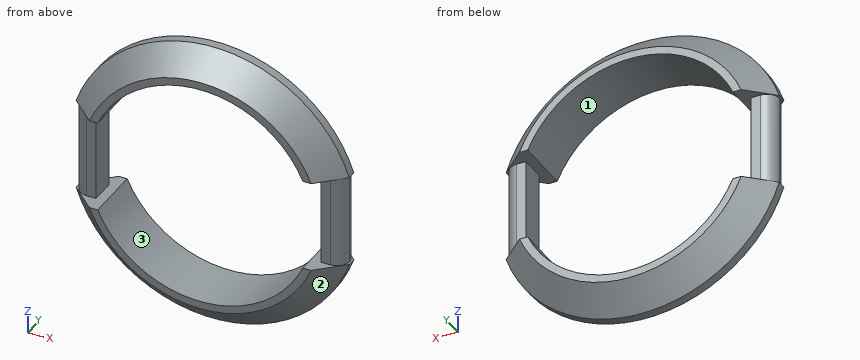
from build123d import *

# Parameters (mm, degrees)
F1_DEPTH      = 2.25
F1_DEPTH_BACK = 2.25
F2_DEPTH      = 1
F2_DEPTH_BACK = 1
F3_T2_ANGLE   = 191.9949180636
F3_T4_ANGLE   = 191.9949180636
F3_T6_ANGLE   = 191.9949180636
F3_T8_ANGLE   = 191.9949180636
F4_T4_DEPTH   = 11.4223278392
F4_T10_DEPTH  = 11.4223278392
F4_T16_DEPTH  = 11.4223278392
F4_T22_DEPTH  = 11.4223278392


# Not quite as in the source:
# - a fillet or chamfer that OpenCascade refuses, or shapes differently, is made with other operations: its cross-section is extruded or revolved along the edge and cut away or added


with BuildPart() as f1:
    # F0 (on Front) → F1 (new body, two sides)
    with BuildSketch(Plane.XZ) as f1_sk:
        with BuildLine():
            ThreePointArc((-8.0962065927, 3.6355279959), (0, 8.875), (8.0962065927, 3.6355279959))
            Line((8.0962065927, 3.6355279959), (8.875, 3.6355279959))
            Line((8.875, 3.6355279959), (10.625, 3.6355279959))
            Line((10.625, 3.6355279959), (10.7783839786, 3.6355279959))
            ThreePointArc((10.7783839786, 3.6355279959), (0, 11.375), (-10.7783839786, 3.6355279959))
            Line((-10.7783839786, 3.6355279959), (-10.625, 3.6355279959))
            Line((-10.625, 3.6355279959), (-8.875, 3.6355279959))
            Line((-8.875, 3.6355279959), (-8.0962065927, 3.6355279959))
        make_face()
    extrude(amount=F1_DEPTH)
    extrude(f1_sk.sketch, amount=-F1_DEPTH_BACK)



with BuildPart() as f1b:
    # F0 (on Front) → F1, piece 2 (new body, two sides)
    with BuildSketch(Plane.XZ) as f1_2_sk:
        with BuildLine():
            Line((8.875, -3.6355279959), (8.0962065927, -3.6355279959))
            ThreePointArc((8.0962065927, -3.6355279959), (0, -8.875), (-8.0962065927, -3.6355279959))
            Line((-8.0962065927, -3.6355279959), (-8.875, -3.6355279959))
            Line((-8.875, -3.6355279959), (-10.625, -3.6355279959))
            Line((-10.625, -3.6355279959), (-10.7783839786, -3.6355279959))
            ThreePointArc((-10.7783839786, -3.6355279959), (0, -11.375), (10.7783839786, -3.6355279959))
            Line((10.7783839786, -3.6355279959), (10.625, -3.6355279959))
            Line((10.625, -3.6355279959), (8.875, -3.6355279959))
        make_face()
    extrude(amount=F1_DEPTH)
    extrude(f1_2_sk.sketch, amount=-F1_DEPTH_BACK)


with BuildPart() as f1_1:
    add(f1.part)

    add(f1b.part)  # F2 merges F1b
    # F0 (on Front) → F2 (join, two sides)
    with BuildSketch(Plane.XZ) as f2_sk:
        Polygon((8.875, 3.6355279959), (8.875, 0), (8.875, -3.6355279959), (10.625, -3.6355279959), (10.625, 3.6355279959), align=None)
        Polygon((-8.875, -3.6355279959), (-8.875, 0), (-8.875, 3.6355279959), (-10.625, 3.6355279959), (-10.625, -3.6355279959), align=None)
    extrude(amount=F2_DEPTH)
    extrude(f2_sk.sketch, amount=-F2_DEPTH_BACK)

    # F3: chamfer of 1.9 on 4 edges, made by hand

    # F3_s1 → F3_t2 (revolve, cut)
    with BuildSketch(Plane(origin=(0, 0, 0), x_dir=(0, 1, 0), z_dir=(-0.1044843578, 0, -0.99452653))):
        Polygon((0.35, 11.375), (2.25, 9.475), (2.25, 11.375), align=None)
    revolve(axis=Axis((0, 2.25, 0), (0, -1, 0)), revolution_arc=F3_T2_ANGLE, mode=Mode.SUBTRACT)

    # F3_s3 → F3_t4 (revolve, cut)
    with BuildSketch(Plane(origin=(0, 0, 0), x_dir=(0, 1, 0), z_dir=(0.1044843578, 0, 0.99452653))):
        Polygon((2.25, 9.475), (0.35, 11.375), (2.25, 11.375), align=None)
    revolve(axis=Axis((0, 2.25, 0), (0, -1, 0)), revolution_arc=F3_T4_ANGLE, mode=Mode.SUBTRACT)

    # F3_s5 → F3_t6 (revolve, cut)
    with BuildSketch(Plane(origin=(0, 0, 0), x_dir=(0, 1, 0), z_dir=(-0.1044843578, 0, -0.99452653))):
        Polygon((-0.35, 11.375), (-2.25, 9.475), (-2.25, 11.375), align=None)
    revolve(axis=Axis((0, -2.25, 0), (0, -1, 0)), revolution_arc=F3_T6_ANGLE, mode=Mode.SUBTRACT)

    # F3_s7 → F3_t8 (revolve, cut)
    with BuildSketch(Plane(origin=(0, 0, 0), x_dir=(0, 1, 0), z_dir=(0.1044843578, 0, 0.99452653))):
        Polygon((-2.25, 9.475), (-0.35, 11.375), (-2.25, 11.375), align=None)
    revolve(axis=Axis((0, -2.25, 0), (0, -1, 0)), revolution_arc=F3_T8_ANGLE, mode=Mode.SUBTRACT)

    # F4: fillet of radius 1 on 4 edges, made by hand


with BuildPart() as f4_tool2:
    # F4_s3 → F4_t4 (new body)
    with BuildSketch(Plane.XY.offset(-5.7111639196)):
        with BuildLine():
            ThreePointArc((10.625, 0), (10.3321067812, -0.7071067812), (9.625, -1))
            Line((9.625, -1), (10.625, -1))
            Line((10.625, -1), (10.625, 0))
        make_face()
    extrude(amount=F4_T4_DEPTH)

    split(bisect_by=Plane.XY.offset(-3.6355279959), keep=Keep.TOP)

    split(bisect_by=Plane.XY.offset(3.6355279959), keep=Keep.BOTTOM)


with BuildPart() as f1_2:
    add(f1_1.part)

    # F4_t1: cut F4_tool2
    add(f4_tool2.part, mode=Mode.SUBTRACT)


with BuildPart() as f4_tool8:
    # F4_s9 → F4_t10 (new body)
    with BuildSketch(Plane.XY.offset(-5.7111639196)):
        with BuildLine():
            ThreePointArc((10.625, 0), (10.3321067812, 0.7071067812), (9.625, 1))
            Line((9.625, 1), (10.625, 1))
            Line((10.625, 1), (10.625, 0))
        make_face()
    extrude(amount=F4_T10_DEPTH)

    split(bisect_by=Plane.XY.offset(-3.6355279959), keep=Keep.TOP)

    split(bisect_by=Plane.XY.offset(3.6355279959), keep=Keep.BOTTOM)


with BuildPart() as f1_3:
    add(f1_2.part)

    # F4_t7: cut F4_tool8
    add(f4_tool8.part, mode=Mode.SUBTRACT)


with BuildPart() as f4_tool14:
    # F4_s15 → F4_t16 (new body)
    with BuildSketch(Plane.XY.offset(5.7111639196)):
        with BuildLine():
            ThreePointArc((-9.625, 1), (-10.3321067812, 0.7071067812), (-10.625, 0))
            Line((-10.625, 0), (-10.625, 1))
            Line((-10.625, 1), (-9.625, 1))
        make_face()
    extrude(amount=-F4_T16_DEPTH)

    split(bisect_by=Plane.XY.offset(-3.6355279959), keep=Keep.TOP)

    split(bisect_by=Plane.XY.offset(3.6355279959), keep=Keep.BOTTOM)


with BuildPart() as f1_4:
    add(f1_3.part)

    # F4_t13: cut F4_tool14
    add(f4_tool14.part, mode=Mode.SUBTRACT)


with BuildPart() as f4_tool20:
    # F4_s21 → F4_t22 (new body)
    with BuildSketch(Plane.XY.offset(5.7111639196)):
        with BuildLine():
            ThreePointArc((-9.625, -1), (-10.3321067812, -0.7071067812), (-10.625, 0))
            Line((-10.625, 0), (-10.625, -1))
            Line((-10.625, -1), (-9.625, -1))
        make_face()
    extrude(amount=-F4_T22_DEPTH)

    split(bisect_by=Plane.XY.offset(-3.6355279959), keep=Keep.TOP)

    split(bisect_by=Plane.XY.offset(3.6355279959), keep=Keep.BOTTOM)


with BuildPart() as f1_5:
    add(f1_4.part)

    # F4_t19: cut F4_tool20
    add(f4_tool20.part, mode=Mode.SUBTRACT)


solid = f1_5.part
Model file for the job. Use its own axes, mm. Face numbers are marked on the shaded views. Coordinates: 2 decimals unless noted, no trailing zeros. Order: outer loops, then holes, each group sorted by start corner. A loop starts at its lowest first (then second) coordinate and runs counter-clockwise, first axis right, second up. Notation, with made-up numbers: (73, -1) -> (77, -1) arc R17 ccw to (77, 31) -> close; hole circle Ø10 at (-25.75, -22). An arc over 180 degrees is marked (long way). Return JSON: item names as keys, results as strings. Group by question number.
Item 1: Wall check: line 1 along Y through (x, z) = (9, 1.5); line 2 along Z through (x, y) = (4.25, -0.75); line 3 along Z through (x, y) = (3, -0.3). Give the ranges that are in metal, low to high. Write a range as [from, to].
Item 2: Saw through at C-C on y = -1.7. Write the cut outline in (x, z) (3 decimals), then the cut area to 3 significant figures.
Item 3: Flat gauge pins, fed straight in: P1, Ø1.5, axis at x = -6.5, y = -1.5, coming from the +Z side; P2, Ø1.3, axis at x = -9, y = 0, coming from the -Z side; P3, Ø2, axis at x = -9.5, y = -1, coming from the +Z side. Where does each tip first touch, or does it go through?
Item 4: Saw through at A-A on z = -2.5. Write the cut outline in (x, y) (3 decimals).
Item 5: Pull direction X, two halves, no side cores. Call the marked faces 1, 2 and 3: pulls with the +X half, pulls with the -X half, needs draft (parallel to the pull), parting line crosses it, or undercut.
Item 6: Saw through at B-B on y = 1.35. Write the cut outline in (x, z) (3 decimals).
Values found:
{
 "1": {"line 1": "y = [-1, 1]", "line 2": "z = [-10.12, -7.79], [7.79, 10.12]", "line 3": "z = [-10.97, -8.35], [8.35, 10.97]"},
 "2": {"outline": "(-9.343, -3.636) arc R10.025 ccw to (9.343, -3.636) -> (8.096, -3.636) arc R8.875 cw to (-8.096, -3.636) -> close; (-9.343, 3.636) -> (-8.096, 3.636) arc R8.875 cw to (8.096, 3.636) -> (9.343, 3.636) arc R10.025 ccw to start", "area": "51.1 mm2"},
 "3": {"P1": "stops at z = 8.99", "P2": "stops at z = -7.72", "P3": "stops at z = 7.28"},
 "4": {"outline": "(-9.625, -1) -> (-8.875, -1) -> (-8.875, 1) -> (-9.625, 1) arc R1 ccw to start; (8.875, -1) -> (9.625, -1) arc R1 ccw to (9.625, 1) -> (8.875, 1) -> close"},
 "5": {"face 1": "undercut", "face 2": "parting line crosses it", "face 3": "undercut"},
 "6": {"outline": "(-9.717, -3.636) arc R10.375 ccw to (9.717, -3.636) -> (8.096, -3.636) arc R8.875 cw to (-8.096, -3.636) -> close; (-9.717, 3.636) -> (-8.096, 3.636) arc R8.875 cw to (8.096, 3.636) -> (9.717, 3.636) arc R10.375 ccw to start"}
}
